Part model, mm, in its own coordinate system. A direction names the side the tool comes from. Give positions to 0.01 mm unless a question says otherwise; leave off trailing zeros. Write each loop counter-clockwise with the first axis right and the second up, starting at its lowest first coordinate (ties: lowest second). Pieces come first, ordered by that corner, then holes. Notation, with made-up numbers: M -5,30 L 54,30 A7 ccw 54,35 Z; hole C 71.5,-22 d9. An arc over 180 degrees is marked long. Answer as CSV lines item,"result". Start each with the question number.
1) Mould opens along Y. For faces 6 (the cylindrical face through (-32, 0, 53)), 7 (the cylindrical face through (-34.01, -14.93, 44.5)), 8 (the flat face through (-34, -22.5, 41)), 9 (the cylindrical face through (1.08, -4.88, 65.87)) say: pulls with the +Y half, pulls with the -Y half, needs draft (parallel to the pull), parting line crosses it, or undercut.
2) Pin check, flat tips, straight feed: pin 1 Ø1.8 at (y, z) = (15, 46) entering from +X; pin 2 Ø12 at (x, y) = (-2, 6) entering from -Z; pin 3 Ø1.5 at (x, z) = (6.5, 56) entering from -Y; pin 4 Ø5 at (y, z) = (15, 22) entering from +X. Stop position of each tip, or through.
3) Tool access for faces 1 (the cylindrical face through (-29.97, 1.32, 87.68)), 2 (the cylindrical face through (-4.336, -19.524, 42.325)), 3 (the flat face through (0, 0, 0)), 4 (the flat face through (-33, 0, 31)), 5 (the cylindrical face through (-34.01, 15.07, 20.5)): list every direction of +Z, -Z, +X, -X, +Y, -Y with a clear straight run to the whole face (end or side of a thin tool).
4) Slice it at A-A, the plane z = 41. Give the cut face in (x, y), plus the area to 3 significant figures.
5) Slice it at C-C, the plane z = 22. Give the cut face in (x, y).
6) Slice it at D-D, the plane x = -23. Give the cut face in (y, z), plus the area to 3 significant figures.
7) Wall check: line 1 along Y through (x, z) = (-34.05, 46); line 2 along Z through (x, y) = (-24, 15); line 3 along Z through (x, y) = (-15, 11.5). Give the ranges that are in metal, low to high. Write a range as from..to.
8) Slice it at B-B, the plane y = 0. Give the cut face in (x, z), plus the area to 3 significant figures.
```python
from build123d import *

# Parameters (mm, degrees)
SKETCH_1_R          = 17.5
EXTRUDE_1_DEPTH     = 30
SKETCH_2_R          = 20
EXTRUDE_2_DEPTH     = 25
SKETCH_3_R          = 5
EXTRUDE_3_DEPTH     = 100
SKETCH_4_R          = 30
EXTRUDE_4_DEPTH     = 25
EXTRUDE_5_DEPTH     = 2
SKETCH_7_W          = 2
SKETCH_7_H          = 45
EXTRUDE_6_DEPTH     = 45
FILLET_3_R          = 5
SKETCH_8_R          = 1.5
CUT_EXTRUDE_1_DEPTH = 5


with BuildPart() as part:
    # 草图1 → 凸台-拉伸1 (new body)
    with BuildSketch(Plane.XY):
        Circle(SKETCH_1_R)
    extrude(amount=EXTRUDE_1_DEPTH)

    # 草图2 → 凸台-拉伸2 (add)
    with BuildSketch(Plane.XY.offset(30)):
        Circle(SKETCH_2_R)
    extrude(amount=EXTRUDE_2_DEPTH)

    # 草图3 → 凸台-拉伸3 (add)
    with BuildSketch(Plane(origin=(0, 0, 0), x_dir=(-1, 0, 0), z_dir=(0, 0, -1))):
        Circle(SKETCH_3_R)
    extrude(amount=-EXTRUDE_3_DEPTH)

    # 草图4 → 凸台-拉伸4 (add)
    with BuildSketch(Plane.XY.offset(100)):
        Circle(SKETCH_4_R)
    extrude(amount=-EXTRUDE_4_DEPTH)

    # 草图6 → 凸台-拉伸5 (add)
    with BuildSketch(Plane.XY.offset(55)):
        with BuildLine():
            Line((0, 22.5), (-35, 22.5))
            Line((-35, 22.5), (-35, -22.5))
            Line((-35, -22.5), (0, -22.5))
            ThreePointArc((0, -22.5), (22.5, 0), (0, 22.5))
        make_face()
    extrude(amount=EXTRUDE_5_DEPTH)

    # 草图7 → 凸台-拉伸6 (add)
    with BuildSketch(Plane.XY.offset(57)):
        with Locations((-34, 0)):
            Rectangle(SKETCH_7_W, SKETCH_7_H)
    extrude(amount=-EXTRUDE_6_DEPTH)

    # 圆角3
    fillet_3_edges = [part.edges().sort_by_distance(p)[0] for p in [
        (-35, 0, 57),
        (-33, 0, 55),
    ]]
    fillet(fillet_3_edges, radius=FILLET_3_R)

    # 草图8 → 切除-拉伸1 (cut)
    with BuildSketch(Plane.ZY.offset(35)):
        with Locations((22, 15)):
            Circle(SKETCH_8_R)
        with Locations((22, -15)):
            Circle(SKETCH_8_R)
        with Locations((46, 15)):
            Circle(SKETCH_8_R)
        with Locations((46, -15)):
            Circle(SKETCH_8_R)
    extrude(amount=-CUT_EXTRUDE_1_DEPTH, mode=Mode.SUBTRACT)


solid = part.part
```
Found:
1,face 6,"needs draft"
1,face 7,"undercut"
1,face 8,"pulls with the -Y half"
1,face 9,"parting line crosses it"
2,pin 1,"x = 14.18"
2,pin 2,"z = 0"
2,pin 3,"y = -21.75"
2,pin 4,"x = 12.25"
3,face 1,"+Z"
3,face 2,"-Z"
3,face 3,"-Z, +X, -X, +Y, -Y"
3,face 4,"-Z, +Y, -Y"
3,face 5,"-X"
4,outline,"M -35,-22.5 L -33,-22.5 L -33,22.5 L -35,22.5 Z; C 0,0 d40"
4,area,"1,350 mm²"
5,outline,"M -35,-22.5 L -33,-22.5 L -33,-16.5 L -35,-16.5 Z; M -35,-13.5 L -33,-13.5 L -33,13.5 L -35,13.5 Z; M -35,16.5 L -33,16.5 L -33,22.5 L -35,22.5 Z; C 0,0 d35"
6,outline,"M -22.5,55 L 22.5,55 L 22.5,57 L -22.5,57 Z; M -19.26,75 L 19.26,75 L 19.26,100 L -19.26,100 Z"
6,area,"1,050 mm²"
7,line 1,"-22.5..-16.5, -13.5..13.5, 16.5..22.5"
7,line 2,"55..57, 75..100"
7,line 3,"30..57, 75..100"
8,outline,"M -35,12 L -33,12 L -33,50 A5 cw -28,55 L -20,55 L -20,30 L -17.5,30 L -17.5,0 L 17.5,0 L 17.5,30 L 20,30 L 20,55 L 22.5,55 L 22.5,57 L 5,57 L 5,75 L 30,75 L 30,100 L -30,100 L -30,75 L -5,75 L -5,57 L -30,57 A5 ccw -35,52 Z"
8,area,"3,930 mm²"
